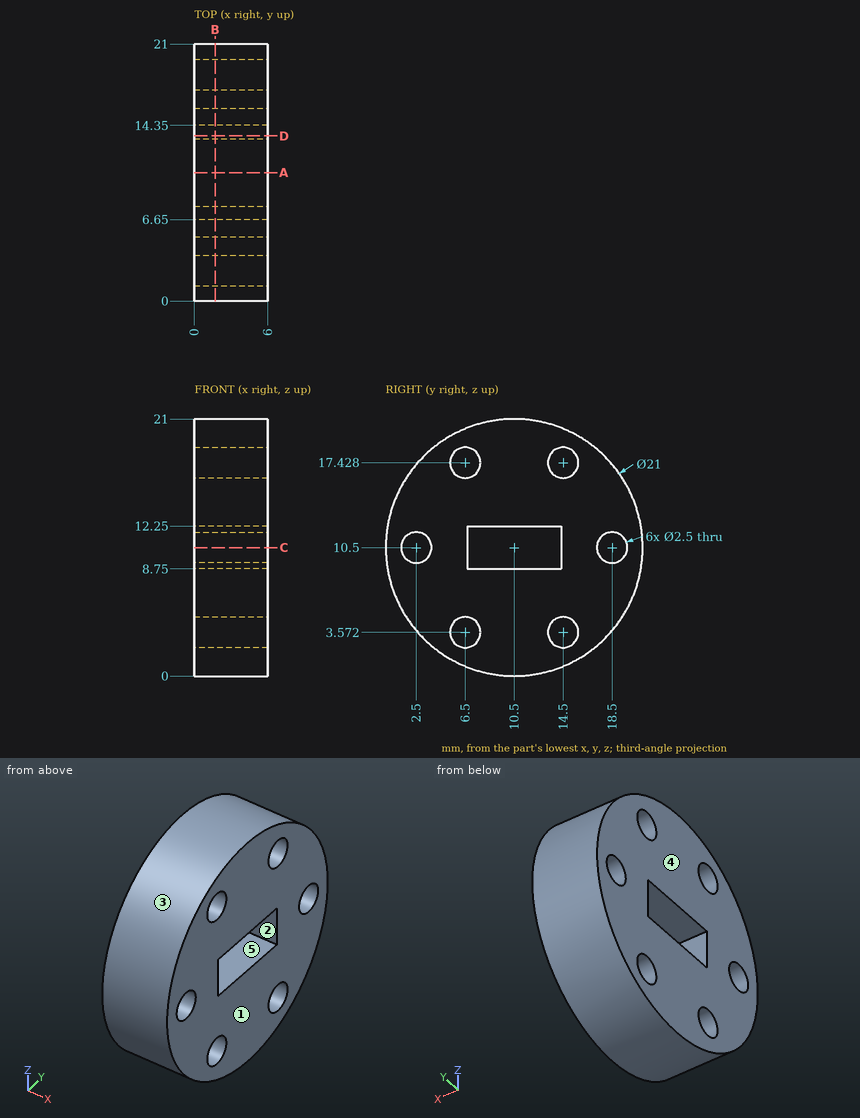
For this review, use the dimensioned drawing (mm, ordinates from the lowest corner) and the shaded views. A direction names the side the tool comes from. Give positions to 0.01 mm unless a question says otherwise; leave off trailing zeros. Write each loop counter-clockwise with the first axis right and the second up, starting at its lowest first coordinate (ties: lowest second). Pieces come first, ordered by that corner, then holes.
(1) To check wall thickness, follow L1, parallel to Y at x = 1.65, z = 10.5; L2, parallel to Z at x = 5.3, y = 9; L3, parallel to Y at x = 5.65, z = 17.25. State the ranges of each line that lie inside material, in increasing order.
(2) Tool access review of the marked faces 4 and 5: name each direction out of +Z, -Z, +X, -X, +Y, -Y from which nothing blocks a thin tool from reaching the whole face with its end or side.
(3) Consider section A-A, the plane y = 10.5. Give the boundary of the cut face in (x, z).
(4) For P1, Ø1.5, axis at x = 3.5, y = 11.5, coming from the +Z side; P2, Ø2, axis at y = 2.5, z = 10.5, coming from the -X side, all flat-tipped, find the tip position at first contact; note any pin that passes through.
(5) Consider section B-B, the plane x = 1.7. Give the boundary of the cut face in (y, z).
(6) Consider section D-D, the plane y = 13.5. Give the boundary of the cut face in (x, z).
(7) The part is to be moulded in two halves that separate along Z. For the marked faces 1, 2 and 3, say which applies: released by +Z, released by -Z, zero draft, split by the parting line, or undercut.
(8) Consider section C-C, the plane z = 10.5. Give the boundary of the cut face in (x, y), and give its area (3 significant figures).
Returned:
1. L1: y = 0 to 1.25, 3.75 to 6.65, 14.35 to 17.25, 19.75 to 21
1. L2: z = 0.11 to 8.75, 12.25 to 20.89
1. L3: y = 2.46 to 5.26, 7.74 to 13.26, 15.74 to 18.54
2. face 4: +Z, -Z, -X, +Y, -Y
2. face 5: +X, -X
3. outline: (0, 0) - (6, 0) - (6, 8.75) - (0, 8.75) - close; (0, 12.25) - (6, 12.25) - (6, 21) - (0, 21) - close
4. P1: stops at z = 21
4. P2: passes through
5. outline: circle Ø21 at (10.5, 10.5); hole circle Ø2.5 at (2.5, 10.5); hole circle Ø2.5 at (6.5, 3.57); hole circle Ø2.5 at (6.5, 17.43); hole (6.65, 8.75) - (14.35, 8.75) - (14.35, 12.25) - (6.65, 12.25) - close; hole circle Ø2.5 at (14.5, 3.57); hole circle Ø2.5 at (14.5, 17.43); hole circle Ø2.5 at (18.5, 10.5)
6. outline: (0, 0.44) - (6, 0.44) - (6, 2.82) - (0, 2.82) - close; (0, 4.32) - (6, 4.32) - (6, 8.75) - (0, 8.75) - close; (0, 12.25) - (6, 12.25) - (6, 16.68) - (0, 16.68) - close; (0, 18.18) - (6, 18.18) - (6, 20.56) - (0, 20.56) - close
7. face 1: zero draft
7. face 2: undercut
7. face 3: split by the parting line
8. outline: (0, 0) - (6, 0) - (6, 1.25) - (0, 1.25) - close; (0, 3.75) - (6, 3.75) - (6, 6.65) - (0, 6.65) - close; (0, 14.35) - (6, 14.35) - (6, 17.25) - (0, 17.25) - close; (0, 19.75) - (6, 19.75) - (6, 21) - (0, 21) - close
8. area: 49.8 mm2
